The model under review builds one solid part; all positions refer to its coordinate system, in mm. A direction names the side the tool comes from. Coordinates: 2 decimals unless noted, no trailing zeros. Order: outer loops, then holes, each group sorted by start corner. A loop starts at its lowest first (then second) coordinate and runs counter-clockwise, first axis right, second up. Notation, with made-up numbers: (-11, -17) -> (45, -17) arc R11 ccw to (45, -5) -> close; hole circle Ø4 at (-20, 16). An arc over 180 degrees is marked (long way). Put each result on its own line as item: value.
Autodesk Fusion 360 part; units mm, degrees
sketch "Sketch1" plane through (0, 0, 0) normal (0, 0, 1) x (1, 0, 0)
  circle A0 centre (0, 0) radius 25
  dimension "d5" = 50
extrude "Extrude1" add sketch "Sketch1" along normal blind 10
sketch "Sketch2" plane through (0, 0, 10) normal (0, 0, 1) x (-1, 0, 0)
  circle A0 centre (0, 0) radius 25
  circle A1 centre (0, 0) radius 22.3
  dimension "d8" = 44.6
extrude "Extrude2" cut sketch "Sketch2" against normal blind 10 contours A1
sketch "Sketch3" plane through (0, 0, 10) normal (0, 0, 1) x (-1, 0, 0)
  circle A0 centre (0, 0) radius 22.3
  circle A1 centre (0, 0) radius 25
  circle A2 centre (0, 0) radius 25
extrude "Extrude3" add sketch "Sketch3" along normal blind 50 contours A0 | A1 A2
sketch "Sketch4" plane through (0, 0, 60) normal (0, 0, 1) x (-1, 0, 0)
  circle A0 centre (0, 0) radius 25
  circle A1 centre (0, 0) radius 20.3
  dimension "d13" = 40.6
extrude "Extrude4" cut sketch "Sketch4" against normal blind 50 contours A1
sketch "Sketch5" plane through (0, 0, 60) normal (0, 0, 1) x (-1, 0, 0)
  circle A0 centre (0, 0) radius 20.3
  circle A1 centre (0, 0) radius 25
  circle A2 centre (0, 0) radius 23.3
  dimension "d16" = 46.6
equation "LowerInnerDiam = 44 mm"
equation "Thickness = 3 mm"
equation "UpperInner = 40 mm"
equation "Tol = 0.6 mm"
equation "d5 = LowerInnerDiam + 2 * Thickness"
equation "d8 = LowerInnerDiam + Tol"
equation "d13 = 40 mm + Tol"
equation "d16 = UpperInner + Tol + 2 * Thickness"
Item 1: Consider section D-D on y = -14.5. Write out the cut boundary in (x, z).
Answers below:
outline: (-20.37, 0) -> (-16.94, 0) -> (-16.94, 10) -> (-14.21, 10) -> (-14.21, 60) -> (-20.37, 60) -> close; (14.21, 10) -> (16.94, 10) -> (16.94, 0) -> (20.37, 0) -> (20.37, 60) -> (14.21, 60) -> close
Item 2: For line 1 (X direction, y = 0, z = 8.25); line 2 (X direction, y = 0, z = 40); line 3 (Z direction, x = 21, y = 5), list the stretches that pass through material, from the lowest coordinate up. Write a range as from..to.
Answers below:
line 1: -25..-22.3, 22.3..25
line 2: -25..-20.3, 20.3..25
line 3: 10..60
Item 3: Mouldability with a two-part tool opening along X and no side actions: class faces 3 (the cylindrical face through (-1.648, 24.946, 29.58)), 4 (the cylindrical face through (-21.27, -6.7, 5.07)), 5 (the flat face through (-22.3, -3.6, 0)) as +X half, -X half, draft (parallel to the pull), parting line (faces both ways), or undercut.
Answers below:
face 3: parting line
face 4: undercut
face 5: draft
Item 4: For faces 1 (the flat face through (0.1, -20.5, 60)), 2 (the flat face through (-5, 20, 10)), list the 3-axis set-ups (+Z, -Z, +X, -X, +Y, -Y) from which the entire face can be reached by the end or side of a thin tool; tool diameter is ignored.
Answers below:
face 1: +Z, +X, -X, +Y, -Y
face 2: -Z
Item 5: For pin 1 Ø10 at (y, z) = (12.5, 6) entering from -X; pin 2 Ø1 at (x, y) = (-17, 11) entering from -Z; pin 3 Ø8 at (y, z) = (6, 30.5) entering from +X, all flat-tipped, find the tip position at first contact; note any pin that passes through.
Answers below:
pin 1: x = -23.85
pin 2: z = 10
pin 3: x = 24.92
Item 6: Consider section A-A on y = -2.5. Write out the cut boundary in (x, z).
Answers below:
outline: (-24.87, 0) -> (-22.16, 0) -> (-22.16, 10) -> (-20.15, 10) -> (-20.15, 60) -> (-24.87, 60) -> close; (20.15, 10) -> (22.16, 10) -> (22.16, 0) -> (24.87, 0) -> (24.87, 60) -> (20.15, 60) -> close
Item 7: Consider section C-C on z = 4. Write out the cut boundary in (x, y).
Answers below:
outline: circle Ø50 at (0, 0); hole circle Ø44.6 at (0, 0)
